Could you check a few things on this drawing? It's one solid part, dimensions in mm from its lowest x, y, z. A direction names the side the tool comes from. Give positions to 0.01 mm unless a question says otherwise; leave off trailing zeros. Order: outer loops, then holes, each group sorted by start corner. A loop starts at its lowest first (then second) coordinate and runs counter-clockwise, first axis right, second up. Notation, with made-up numbers: (-13, 77.25) - (35, 77.25) arc R33 cw to (35, 106.25) - close; hole circle Ø8 at (-27.75, 67). An arc over 180 degrees is marked (long way). Return JSON: item names as keys, results as strings.
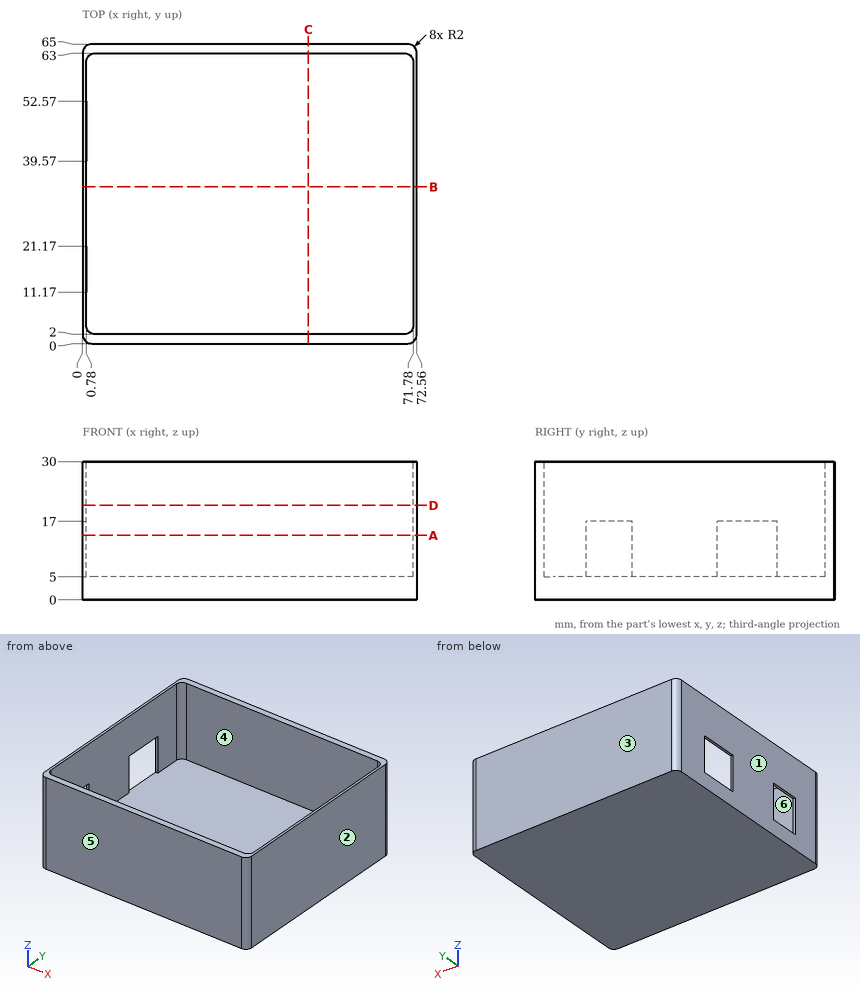
1. Suppose I cut it at A-A (z = 14). List the corners of the cut face in (x, y) for me.
Checks:
{"outline": "(0, 2) arc R2 ccw to (2, 0) - (70.56, 0) arc R2 ccw to (72.56, 2) - (72.56, 63) arc R2 ccw to (70.56, 65) - (2, 65) arc R2 ccw to (0, 63) - (0, 52.57) - (0.78, 52.57) - (0.78, 61) arc R2 cw to (2.78, 63) - (69.78, 63) arc R2 cw to (71.78, 61) - (71.78, 4) arc R2 cw to (69.78, 2) - (2.78, 2) arc R2 cw to (0.78, 4) - (0.78, 11.17) - (0, 11.17) - close; (0, 21.17) - (0.78, 21.17) - (0.78, 39.57) - (0, 39.57) - close"}
2. For pin 1 Ø0.9 at (x, z) = (0.5, 9) entering from +Y; pin 2 Ø3 at (y, z) = (16, 14.5) entering from -X, each with a flat end and sliding along its axis, tell me the tip position at first contact or that it passes through.
Checks:
{"pin 1": "y = 64.7", "pin 2": "x = 71.78"}
3. Suppose I cut it at B-B (y = 34). List the corners of the cut face in (x, z) for me.
Checks:
{"outline": "(0, 0) - (72.56, 0) - (72.56, 30) - (71.78, 30) - (71.78, 5) - (0.78, 5) - (0.78, 30) - (0, 30) - close"}
4. Suppose I cut it at D-D (z = 20.5). List the corners of the cut face in (x, y) for me, plus the area to 3 significant figures.
Checks:
{"outline": "(0, 2) arc R2 ccw to (2, 0) - (70.56, 0) arc R2 ccw to (72.56, 2) - (72.56, 63) arc R2 ccw to (70.56, 65) - (2, 65) arc R2 ccw to (0, 63) - close; hole (0.78, 4) arc R2 ccw to (2.78, 2) - (69.78, 2) arc R2 ccw to (71.78, 4) - (71.78, 61) arc R2 ccw to (69.78, 63) - (2.78, 63) arc R2 ccw to (0.78, 61) - close", "area": "385 mm^2"}
5. If I drill on L1, parallel to X at y = 29, z = 28.75; L2, parallel to Y at x = 33.5, z = 16.75; L3, parallel to Z at x = 46, y = 13.5, over which ranges is the centre line in solid material (lowest first)? Write a range as [from, to].
Checks:
{"L1": "[0, 0.78], [71.78, 72.56]", "L2": "[0, 2], [63, 65]", "L3": "[0, 5]"}
6. Suppose I cut it at C-C (x = 49). List the corners of the cut face in (y, z) for me.
Checks:
{"outline": "(0, 0) - (65, 0) - (65, 30) - (63, 30) - (63, 5) - (2, 5) - (2, 30) - (0, 30) - close"}
7. On a 3-axis mill with a long thin cutter (end or side, diameter ignored), from which of +Z, -Z, +X, -X, +Y, -Y can I reach the whole of each face in a straight line? I mean the marked faces 5 and 6. Say none if no direction works.
Checks:
{"face 5": "+Z, -Z, +X, -X, -Y", "face 6": "+Z"}
8. Thinking about a two-plate mould opening in X: for the marked faces 1, 2, 3 and 4, which applies, +X half, -X half, draft (parallel to the pull), parting line (faces both ways), or undercut?
Checks:
{"face 1": "-X half", "face 2": "+X half", "face 3": "draft", "face 4": "undercut"}
